```python
from build123d import *

# Parameters (mm, degrees)
ESTRUSIONE_ESTRUSIONE1_DEPTH             = 100
TAGLIO_ESTRUSIONE5_DEPTH                 = 704.628710974
TAGLIO_ESTRUSIONE5_DEPTH_BACK            = 704.628710974
SCHIZZO2_R                               = 15
TAGLIO_ESTRUSIONE6_DEPTH                 = 704.628710974
TAGLIO_ESTRUSIONE6_DEPTH_BACK            = 704.628710974
SCHIZZO3_W                               = 85
SCHIZZO3_H                               = 100
ESTRUSIONE_ESTRUSIONE2_REACH             = 705.629
SCHIZZO4_W                               = 50
SCHIZZO4_H                               = 50
ESTRUSIONE_ESTRUSIONE2_DIRECTION_2_REACH = 705.629


with BuildPart() as part:
    # Schizzo1 → Estrusione-Estrusione1 (new body)
    with BuildSketch(Plane(origin=(0, 0, 0), x_dir=(1, 0, 0), z_dir=(0, 1, 0))):
        Polygon((-332.846822006, -200), (-332.846822006, 200), (667.153177994, 200), (667.153177994, 120), (-232.846822006, 120), (-232.846822006, -120), (667.153177994, -120), (667.153177994, -200), align=None)
    extrude(amount=ESTRUSIONE_ESTRUSIONE1_DEPTH)

    # Schizzo2 → Taglio-Estrusione5 (cut, two sides: drawn at the far end of the back side and taken through both)
    with BuildSketch(Plane.XY.offset(-TAGLIO_ESTRUSIONE5_DEPTH_BACK)):
        with Locations((-315.846822006, 50)):
            Circle(SCHIZZO2_R)
        with Locations((-59.546822006, 50)):
            Circle(SCHIZZO2_R)
        with Locations((540.453177994, 50)):
            Circle(SCHIZZO2_R)
    extrude(amount=TAGLIO_ESTRUSIONE5_DEPTH + TAGLIO_ESTRUSIONE5_DEPTH_BACK, mode=Mode.SUBTRACT)

    # Schizzo3 → Taglio-Estrusione6 (cut, two sides: drawn at the far end of the back side and taken through both)
    with BuildSketch(Plane(origin=(0, 0, 0), x_dir=(1, 0, 0), z_dir=(0, 1, 0)).offset(-TAGLIO_ESTRUSIONE6_DEPTH_BACK)):
        with Locations((-290.346822006, 0)):
            Rectangle(SCHIZZO3_W, SCHIZZO3_H)
    extrude(amount=TAGLIO_ESTRUSIONE6_DEPTH + TAGLIO_ESTRUSIONE6_DEPTH_BACK, mode=Mode.SUBTRACT)

    # Schizzo4 → Estrusione-Estrusione2 (add, up to next)
    with BuildSketch(Plane.XY, mode=Mode.PRIVATE) as estrusione_estrusione2_sk1:
        with Locations((-5, 50)):
            Rectangle(SCHIZZO4_W, SCHIZZO4_H)
    estrusione_estrusione2_tool1 = extrude(estrusione_estrusione2_sk1.sketch, amount=ESTRUSIONE_ESTRUSIONE2_REACH, mode=Mode.PRIVATE) - part.part
    add(estrusione_estrusione2_tool1.solids().sort_by_distance((-5, 50, 0))[0])

    # Schizzo4 → Estrusione-Estrusione2 direction 2 (add, up to next)
    with BuildSketch(Plane.XY, mode=Mode.PRIVATE) as estrusione_estrusione2_direction_2_sk1:
        with Locations((-5, 50)):
            Rectangle(SCHIZZO4_W, SCHIZZO4_H)
    estrusione_estrusione2_direction_2_tool1 = extrude(estrusione_estrusione2_direction_2_sk1.sketch, amount=-ESTRUSIONE_ESTRUSIONE2_DIRECTION_2_REACH, mode=Mode.PRIVATE) - part.part
    add(estrusione_estrusione2_direction_2_tool1.solids().sort_by_distance((-5, 50, 0))[0])


solid = part.part
```
Verification items for the finished model (mm, model axes). A direction names the side the tool comes from. Round coordinates to 2 decimals unless told otherwise and drop trailing zeros. Write each loop counter-clockwise with the first axis right and the second up, starting at its lowest first coordinate (ties: lowest second). Pieces come first, ordered by that corner, then holes.
1. Draft check along Z on faces 6 (the flat face through (-291, 49, -50)), 7 (the flat face through (160, 49, -200)), 8 (the flat face through (174, 49, 200)), 9 (the flat face through (174, 0, -136)). Enter one of: +Z half, -Z half, draft (parallel to the pull), parting line (faces both ways), or undercut.
2. Access from +Z, -Z, +X, -X, +Y, -Y to the whole of each face (thin tool, end or side, straight path). Record for faces 1 (the flat face through (-247.847, 49, 1)), 2 (the flat face through (20, 50, 2)), 3 (the flat face through (-30, 50, 2)), 4 (the flat face through (-5, 75, 2)), 5 (the flat face through (-5, 25, 2)).
3. Section check D-D on z = 143. Enter the section's corners in (x, y).
4. Gauge pin test, flat ends, axial feed: P1, Ø1.5, axis at y = 44.5, z = 39.5, coming from the +X side; P2, Ø25, axis at x = -14, z = -39.5, coming from the -Y side; P3, Ø15, axis at x = 4.5, z = -35.5, coming from the +Y side. Record the tip position at first contact, or that the pin passes through.
5. Section check C-C on y = 90. Enter the section's corners in (x, z).
6. Scan lines: L1, parallel to X at y = 50, z = 149; L2, parallel to X at y = 49, z = 113; L3, parallel to Z at x = -141.5, y = 58. Record each from-to range of solid material in increasing order.
7. Section check A-A on z = -95.5. Enter the section's corners in (x, y), plus the area to 3 significant figures.
8. Section check B-B on x = 61.5. Enter the section's corners in (y, z).
Answer:
1. face 6: undercut
1. face 7: -Z half
1. face 8: +Z half
1. face 9: draft
2. face 1: -X, +Y, -Y
2. face 2: +X, +Y, -Y
2. face 3: +Y, -Y
2. face 4: +X, +Y
2. face 5: +X, -Y
3. outline: (-332.85, 0) - (667.15, 0) - (667.15, 100) - (-332.85, 100) - close; hole circle Ø30 at (-315.85, 50); hole circle Ø30 at (-59.55, 50); hole circle Ø30 at (540.45, 50)
4. P1: stops at x = 20
4. P2: stops at y = 25
4. P3: stops at y = 75
5. outline: (-332.85, -200) - (667.15, -200) - (667.15, -120) - (-232.85, -120) - (-232.85, 120) - (667.15, 120) - (667.15, 200) - (-332.85, 200) - (-332.85, 50) - (-247.85, 50) - (-247.85, -50) - (-332.85, -50) - close
6. L1: x = -332.85 to -330.85, -300.85 to -74.55, -44.55 to 525.45, 555.45 to 667.15
6. L2: x = -332.85 to -330.81, -300.88 to -232.85, -30 to 20
6. L3: z = -200 to -120, 120 to 200
7. outline: (-332.85, 0) - (-232.85, 0) - (-232.85, 100) - (-332.85, 100) - close; (-30, 25) - (20, 25) - (20, 75) - (-30, 75) - close; hole circle Ø30 at (-315.85, 50)
7. area: 11,800 mm2
8. outline: (0, -200) - (100, -200) - (100, -120) - (0, -120) - close; (0, 120) - (100, 120) - (100, 200) - (0, 200) - close
